from build123d import *

# Parameters (mm, degrees)
SKETCH1_W           = 98
SKETCH1_H           = 30
SKETCH1_R           = 7
SKETCH1_R_2         = 1
BOSS_EXTRUDE1_DEPTH = 5.9
SKETCH3_W           = 5.9
SKETCH3_H           = 10
CUT_EXTRUDE2_DEPTH  = 10
SKETCH4_R           = 7
SKETCH4_R_2         = 1
CUT_EXTRUDE3_DEPTH  = 10
FILLET1_R           = 10
CUT_EXTRUDE4_REACH  = 7.9
SKETCH5_R           = 2.05
SKETCH6_R           = 2.05
CUT_EXTRUDE5_DEPTH  = 10


with BuildPart() as part:
    # Sketch1 → Boss-Extrude1 (new body)
    with BuildSketch(Plane(origin=(0, 0, 0), x_dir=(1, 0, 0), z_dir=(0, 1, 0))):
        Rectangle(SKETCH1_W, SKETCH1_H)
        with Locations((-34, 0)):
            Circle(SKETCH1_R, mode=Mode.SUBTRACT)
        with Locations((-44.4, 0)):
            Circle(SKETCH1_R_2, mode=Mode.SUBTRACT)
        with Locations((-47.4, 0)):
            Circle(SKETCH1_R_2, mode=Mode.SUBTRACT)
        with Locations((-34, 10.4)):
            Circle(SKETCH1_R_2, mode=Mode.SUBTRACT)
        with Locations((-34, 13.4)):
            Circle(SKETCH1_R_2, mode=Mode.SUBTRACT)
        with Locations((-23.6, 0)):
            Circle(SKETCH1_R_2, mode=Mode.SUBTRACT)
        with Locations((-20.6, 0)):
            Circle(SKETCH1_R_2, mode=Mode.SUBTRACT)
        with Locations((-34, -10.4)):
            Circle(SKETCH1_R_2, mode=Mode.SUBTRACT)
        with Locations((-34, -13.4)):
            Circle(SKETCH1_R_2, mode=Mode.SUBTRACT)
    extrude(amount=BOSS_EXTRUDE1_DEPTH)

    # Sketch3 → Cut-Extrude2 (cut)
    with BuildSketch(Plane(origin=(0, 5.9, 0), x_dir=(1, 0, 0), z_dir=(0, 1, 0))):
        with Locations((-6.05, 0)):
            Rectangle(SKETCH3_W, SKETCH3_H)
    extrude(amount=-CUT_EXTRUDE2_DEPTH, mode=Mode.SUBTRACT)

    # Sketch4 → Cut-Extrude3 (cut)
    with BuildSketch(Plane(origin=(0, 5.9, 0), x_dir=(1, 0, 0), z_dir=(0, 1, 0))):
        with Locations((-34, 0)):
            Circle(SKETCH4_R)
        with Locations((-34, -13.4)):
            Circle(SKETCH4_R_2)
        with Locations((-34, -10.4)):
            Circle(SKETCH4_R_2)
        with Locations((-44.4, 0)):
            Circle(SKETCH4_R_2)
        with Locations((-47.4, 0)):
            Circle(SKETCH4_R_2)
        with Locations((-34, 13.4)):
            Circle(SKETCH4_R_2)
        with Locations((-23.6, 0)):
            Circle(SKETCH4_R_2)
        with Locations((-20.6, 0)):
            Circle(SKETCH4_R_2)
        with Locations((-34, 10.4)):
            Circle(SKETCH4_R_2)
        with Locations((29, -13.4)):
            Circle(SKETCH4_R_2)
        with Locations((29, -10.4)):
            Circle(SKETCH4_R_2)
        with Locations((42.4, 0)):
            Circle(SKETCH4_R_2)
        with Locations((39.4, 0)):
            Circle(SKETCH4_R_2)
        with Locations((29, 0)):
            Circle(SKETCH4_R)
        with Locations((29, 10.4)):
            Circle(SKETCH4_R_2)
        with Locations((29, 13.4)):
            Circle(SKETCH4_R_2)
        with Locations((18.6, 0)):
            Circle(SKETCH4_R_2)
        with Locations((15.6, 0)):
            Circle(SKETCH4_R_2)
    extrude(amount=-CUT_EXTRUDE3_DEPTH, mode=Mode.SUBTRACT)

    # Fillet1
    fillet1_edges = [part.edges().sort_by_distance(p)[0] for p in [
        (49, 2.95, 15),
        (-49, 2.95, 15),
        (-49, 2.95, -15),
        (49, 2.95, -15),
    ]]
    fillet(fillet1_edges, radius=FILLET1_R)

    # Sketch5 → Cut-Extrude4 (cut, up to next)
    with BuildSketch(Plane(origin=(0, 5.9, 0), x_dir=(1, 0, 0), z_dir=(0, 1, 0)), mode=Mode.PRIVATE) as cut_extrude4_sk1:
        with Locations((-9, 5)):
            Circle(SKETCH5_R)
    cut_extrude4_tool1 = extrude(cut_extrude4_sk1.sketch, amount=-CUT_EXTRUDE4_REACH, mode=Mode.PRIVATE) & part.part
    add(cut_extrude4_tool1.solids().sort_by_distance((-9, 5.9, -5))[0], mode=Mode.SUBTRACT)
    # Sketch5 → Cut-Extrude4 (cut, up to next)
    with BuildSketch(Plane(origin=(0, 5.9, 0), x_dir=(1, 0, 0), z_dir=(0, 1, 0)), mode=Mode.PRIVATE) as cut_extrude4_sk2:
        with Locations((-3.1, 5)):
            Circle(SKETCH5_R)
    cut_extrude4_tool2 = extrude(cut_extrude4_sk2.sketch, amount=-CUT_EXTRUDE4_REACH, mode=Mode.PRIVATE) & part.part
    add(cut_extrude4_tool2.solids().sort_by_distance((-3.1, 5.9, -5))[0], mode=Mode.SUBTRACT)
    # Sketch5 → Cut-Extrude4 (cut, up to next)
    with BuildSketch(Plane(origin=(0, 5.9, 0), x_dir=(1, 0, 0), z_dir=(0, 1, 0)), mode=Mode.PRIVATE) as cut_extrude4_sk3:
        with Locations((-3.1, -5)):
            Circle(SKETCH5_R)
    cut_extrude4_tool3 = extrude(cut_extrude4_sk3.sketch, amount=-CUT_EXTRUDE4_REACH, mode=Mode.PRIVATE) & part.part
    add(cut_extrude4_tool3.solids().sort_by_distance((-3.1, 5.9, 5))[0], mode=Mode.SUBTRACT)
    # Sketch5 → Cut-Extrude4 (cut, up to next)
    with BuildSketch(Plane(origin=(0, 5.9, 0), x_dir=(1, 0, 0), z_dir=(0, 1, 0)), mode=Mode.PRIVATE) as cut_extrude4_sk4:
        with Locations((-9, -5)):
            Circle(SKETCH5_R)
    cut_extrude4_tool4 = extrude(cut_extrude4_sk4.sketch, amount=-CUT_EXTRUDE4_REACH, mode=Mode.PRIVATE) & part.part
    add(cut_extrude4_tool4.solids().sort_by_distance((-9, 5.9, 5))[0], mode=Mode.SUBTRACT)

    # Sketch6 → Cut-Extrude5 (cut)
    with BuildSketch(Plane(origin=(0, 5.9, 0), x_dir=(1, 0, 0), z_dir=(0, 1, 0))):
        with Locations((-17.05, 10)):
            Circle(SKETCH6_R)
        with Locations((-17.05, -10)):
            Circle(SKETCH6_R)
        with Locations((4.95, -10)):
            Circle(SKETCH6_R)
        with Locations((4.95, 10)):
            Circle(SKETCH6_R)
    extrude(amount=-CUT_EXTRUDE5_DEPTH, mode=Mode.SUBTRACT)


solid = part.part
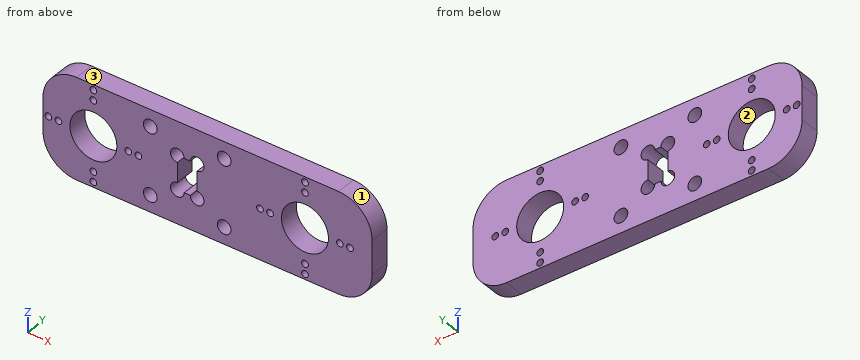
The model under review builds one solid part; all positions refer to its coordinate system, in mm. Face numbers are marked on the shaded views. Round coordinates to 2 decimals unless told otherwise and drop trailing zeros. Loops run counter-clockwise (first coordinate to the right, second up) from the corner with the lowest first, then second, coordinate; pieces in that order, holes last. Notation, with made-up numbers: (-7.75, 36.5) -> (43.25, 36.5) arc R26 cw to (43.25, 62.5) -> close; hole circle Ø9 at (-27, 78.25). An arc over 180 degrees is marked (long way). Write item = value, one per line. Start each with the question number.
Item 1: Take a section at C-C on z = 2. Give the boundary of the cut face in (x, y).
Item 2: Take a section at B-B on x = 15.6. Give the boundary of the cut face in (y, z).
Item 3: Take a section at A-A on x = 29. Give the boundary of the cut face in (y, z).
Item 4: Insertion check: pin 1 (4.5 mm diameter, centred on x = -9, z = 5, fed in from +Y). The pin has a flat end and moves straight along its axis. Give the tip position at first contact, or say it passes through.
Item 5: Mouldability with a two-part tool opening along X and no side actions: class the marked faces 1, 2 and 3 as released by +X, released by -X, zero draft, split by the parting line, or undercut.
Item 6: To check wall thickness, follow L1, parallel to X at y = 4.8, z = -1.5; L2, parallel to X at y = 3.7, z = -10.4; L3, parallel to Z at x = -15.5, y = 4.45. State the ranges of each line that lie inside material, in increasing order.
Item 7: Take a section at D-D on z = 13.4. Give the boundary of the cut face in (x, y).
Result:
q1.outline = (-49, 0) -> (-40.71, 0) -> (-40.71, 5.9) -> (-49, 5.9) -> close; (-27.29, 0) -> (-9, 0) -> (-9, 5.9) -> (-27.29, 5.9) -> close; (-3.1, 0) -> (22.29, 0) -> (22.29, 5.9) -> (-3.1, 5.9) -> close; (35.71, 0) -> (49, 0) -> (49, 5.9) -> (35.71, 5.9) -> close
q2.outline = (0, -15) -> (5.9, -15) -> (5.9, -1) -> (0, -1) -> close; (0, 1) -> (5.9, 1) -> (5.9, 15) -> (0, 15) -> close
q3.outline = (0, -15) -> (5.9, -15) -> (5.9, -14.4) -> (0, -14.4) -> close; (0, -12.4) -> (5.9, -12.4) -> (5.9, -11.4) -> (0, -11.4) -> close; (0, -9.4) -> (5.9, -9.4) -> (5.9, -7) -> (0, -7) -> close; (0, 7) -> (5.9, 7) -> (5.9, 9.4) -> (0, 9.4) -> close; (0, 11.4) -> (5.9, 11.4) -> (5.9, 12.4) -> (0, 12.4) -> close; (0, 14.4) -> (5.9, 14.4) -> (5.9, 15) -> (0, 15) -> close
q4.pin_1 = 5.9
q5.face_1 = released by +X
q5.face_2 = undercut
q5.face_3 = zero draft
q6.L1 = -49 to -40.84, -27.16 to -9, -3.1 to 22.16, 35.84 to 49
q6.L2 = -47.42 to -35, -33 to -19.06, -15.04 to 2.94, 6.96 to 28, 30 to 47.42
q6.L3 = -15 to -11.34, -8.66 to 8.66, 11.34 to 15
q7.outline = (-44.43, 0) -> (-35, 0) -> (-35, 5.9) -> (-44.43, 5.9) -> close; (-33, 0) -> (28, 0) -> (28, 5.9) -> (-33, 5.9) -> close; (30, 0) -> (44.43, 0) -> (44.43, 5.9) -> (30, 5.9) -> close
